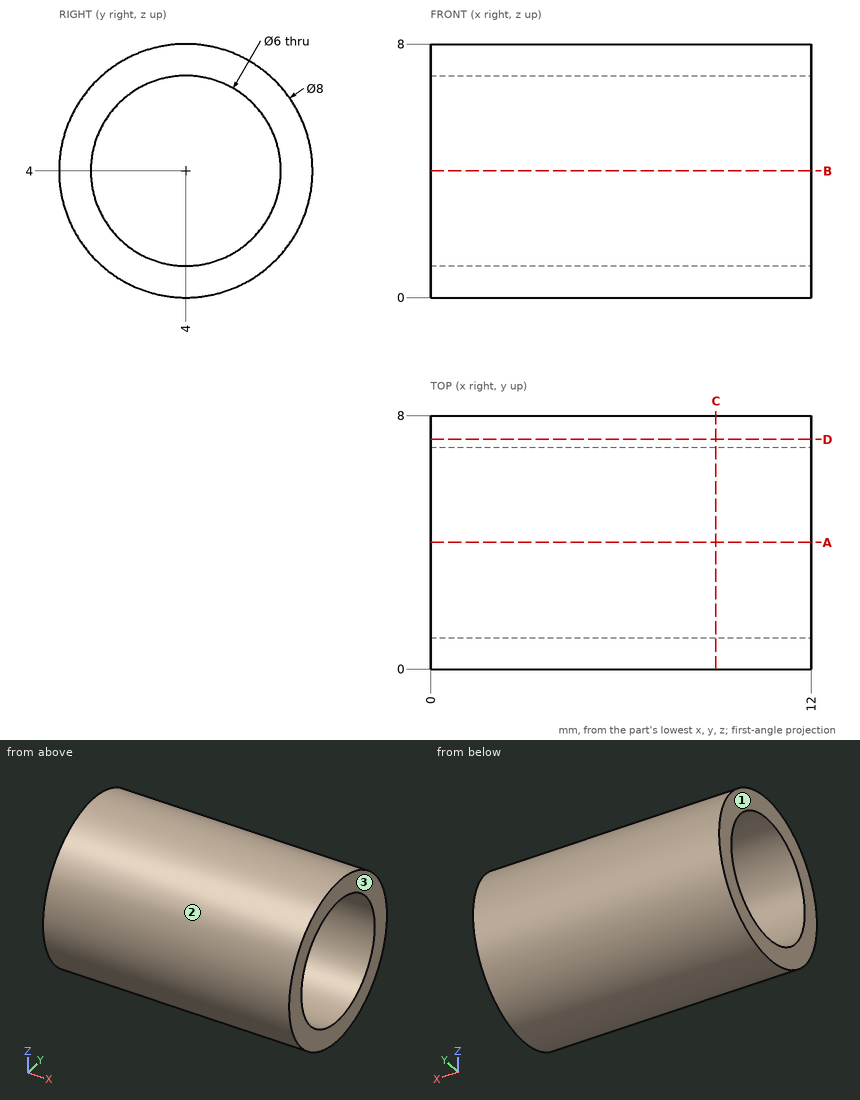
Geometry check sheet. Reference: drawing and pictorial views, mm from the part's lowest x, y, z. Give positions to 0.01 mm unless a question says otherwise; leave off trailing zeros. Order: outer loops, then holes, each group sorted by start corner. A loop starts at its lowest first (then second) coordinate and runs counter-clockwise, first axis right, second up. Notation, with made-up numbers: M 77.25,7 L 96.25,7 A17 cw 96.25,11 Z; hole C 47,-17 d11. An arc over 180 degrees is marked long. Return JSON: item names as keys, results as strings. Group by question number.
1) Go/stop test with flat-tipped pins: pin 1 Ø1.5 at (x, y) = (7.5, 5) entering from +Z; pin 2 Ø2 at (x, y) = (2.5, 6.5) entering from +Z. Record where each tip stops, or that it passes through.
2) Mould release check, pull along X, two halves, no side actions. Record for the marked faces 1, 2 and 3: pulls with the +X half, pulls with the -X half, needs draft (parallel to the pull), parting line crosses it, or undercut.
3) Scan lines: line 1 (Z direction, x = 9.5, y = 4); line 2 (Y direction, x = 2, z = 5.75); line 3 (Z direction, x = 2.5, y = 6). Record each from-to range of solid material in increasing order.
4) Section check A-A on y = 4. Record the cut outline in (x, z), and give its area (3 significant figures).
5) Section check C-C on x = 9. Record the cut outline in (y, z).
6) Section check D-D on y = 7.25. Record the cut outline in (x, z), and give its area (3 significant figures).
Answer block:
{
 "1": {"pin 1": "stops at z = 7.99", "pin 2": "stops at z = 7.71"},
 "2": {"face 1": "pulls with the -X half", "face 2": "needs draft", "face 3": "pulls with the +X half"},
 "3": {"line 1": "z = 0 to 1, 7 to 8", "line 2": "y = 0.4 to 1.56, 6.44 to 7.6", "line 3": "z = 0.54 to 1.76, 6.24 to 7.46"},
 "4": {"outline": "M 0,0 L 12,0 L 12,1 L 0,1 Z; M 0,7 L 12,7 L 12,8 L 0,8 Z", "area": "24.0 mm^2"},
 "5": {"outline": "C 4,4 d8; hole C 4,4 d6"},
 "6": {"outline": "M 0,1.67 L 12,1.67 L 12,6.33 L 0,6.33 Z", "area": "56.0 mm^2"}
}
